Verification items for the finished model (mm, model axes). A direction names the side the tool comes from. Give positions to 0.01 mm unless a question says otherwise; leave off trailing zeros. Loops run counter-clockwise (first coordinate to the right, second up) from the corner with the lowest first, then second, coordinate; pieces in that order, holes last. Notation, with made-up numbers: (-30.5, -21) - (-14.5, -21) arc R9 ccw to (-14.5, -10) - close; hole circle Ø4 at (-7.5, -9.75). An arc over 180 degrees is marked (long way). Answer in a Markdown table with one row per item.
```python
from build123d import *

# Parameters (mm, degrees)
ESBO_O1_W                = 100
ESBO_O1_H                = 50
ESBO_O1_R                = 1
RESSALTO_EXTRUS_O1_DEPTH = 1.5
ESBO_O2_R                = 8.5
ESBO_O2_W                = 53
ESBO_O2_H                = 21
ESBO_O2_W_2              = 6
ESBO_O2_H_2              = 6
ESBO_O2_W_3              = 26.2
ESBO_O2_H_3              = 26.3
RESSALTO_EXTRUS_O4_DEPTH = 14.7
ESBO_O3_W                = 22.891769865
ESBO_O3_H                = 8.050029258
CORTE_EXTRUS_O1_DEPTH    = 9.7
ESBO_O4_R                = 3.5
RESSALTO_EXTRUS_O5_DEPTH = 17
ESBO_O5_W                = 55.7
ESBO_O5_H                = 43
RESSALTO_EXTRUS_O6_DEPTH = 18
ESBO_O6_W                = 26.2
ESBO_O6_H                = 14
RESSALTO_EXTRUS_O7_DEPTH = 0.2
ESBO_O7_W                = 26.2
ESBO_O7_H                = 10.560021921
CORTE_EXTRUS_O2_DEPTH    = 20.2


with BuildPart() as part:
    # Esboço1 → Ressalto-extrusão1 (new body)
    with BuildSketch(Plane(origin=(0, 0, 0), x_dir=(1, 0, 0), z_dir=(0, 1, 0))):
        Rectangle(ESBO_O1_W, ESBO_O1_H)
        with Locations(Location((43.75, 18.75, 0), (0, 0, 270))):
            Circle(ESBO_O1_R, mode=Mode.SUBTRACT)
        with Locations(Location((43.75, -18.75, 0), (0, 0, 270))):
            Circle(ESBO_O1_R, mode=Mode.SUBTRACT)
        with Locations(Location((-43.75, 18.749999801, 0), (0, 0, 270))):
            Circle(ESBO_O1_R, mode=Mode.SUBTRACT)
        with Locations(Location((-43.751173924, -18.750000181, 0), (0, 0, 270))):
            Circle(ESBO_O1_R, mode=Mode.SUBTRACT)
    extrude(amount=RESSALTO_EXTRUS_O1_DEPTH)

    # Esboço2 → Ressalto-extrusão4 (add)
    with BuildSketch(Plane(origin=(0, 1.5, 0), x_dir=(1, 0, 0), z_dir=(0, 1, 0))):
        with Locations(Location((33.5, -22.5, 0), (0, 0, 342.895364823))):
            Circle(ESBO_O2_R)
        with Locations(Location((-34.1, -22.5, 0), (0, 0, 197.104635177))):
            Circle(ESBO_O2_R)
        with Locations((-15.9, 5.5)):
            Rectangle(ESBO_O2_W, ESBO_O2_H)
        with Locations((22.3, 13)):
            Rectangle(ESBO_O2_W_2, ESBO_O2_H_2)
        with Locations((35.6, 13)):
            Rectangle(ESBO_O2_W_2, ESBO_O2_H_2)
        with Locations((-0.1, -19.15)):
            Rectangle(ESBO_O2_W_3, ESBO_O2_H_3)
    extrude(amount=RESSALTO_EXTRUS_O4_DEPTH)

    # Esboço3 → Corte-extrusão1 (cut)
    with BuildSketch(Plane(origin=(0, 16.2, 0), x_dir=(1, 0, 0), z_dir=(0, 1, 0))):
        with Locations((27.154115068, 14.025014629)):
            Rectangle(ESBO_O3_W, ESBO_O3_H)
    extrude(amount=-CORTE_EXTRUS_O1_DEPTH, mode=Mode.SUBTRACT)

    # Esboço4 → Ressalto-extrusão5 (add)
    with BuildSketch(Plane(origin=(0, 16.2, 0), x_dir=(1, 0, 0), z_dir=(0, 1, 0))):
        with Locations(Location((33.5, -22.5, 0), (0, 0, 270))):
            Circle(ESBO_O4_R)
        with Locations(Location((-34.1, -22.5, 0), (0, 0, 270))):
            Circle(ESBO_O4_R)
    extrude(amount=RESSALTO_EXTRUS_O5_DEPTH)

    # Esboço5 → Ressalto-extrusão6 (add)
    with BuildSketch(Plane.XZ):
        with Locations((-4.35, -5.5)):
            Rectangle(ESBO_O5_W, ESBO_O5_H)
    extrude(amount=RESSALTO_EXTRUS_O6_DEPTH)

    # Esboço6 → Ressalto-extrusão7 (add)
    with BuildSketch(Plane(origin=(0, 16.2, 0), x_dir=(1, 0, 0), z_dir=(0, 1, 0))):
        with Locations((-0.1, -17)):
            Rectangle(ESBO_O6_W, ESBO_O6_H)
    extrude(amount=RESSALTO_EXTRUS_O7_DEPTH)

    # Esboço7 → Corte-extrusão2 (cut)
    with BuildSketch(Plane.XY.offset(32.3)):
        with Locations((-0.1, 6.780010961)):
            Rectangle(ESBO_O7_W, ESBO_O7_H)
    extrude(amount=-CORTE_EXTRUS_O2_DEPTH, mode=Mode.SUBTRACT)


solid = part.part
```
Q1. Draft check along X on faces 6 (the face through (-16, 16.2, -6)), 7 (the face through (42, 8.7, 22.4)), 8 (the face through (-32.2, -9, -6)). Enter one of: +X half, -X half, draft (parallel to the pull), parting line (faces both ways), or undercut.
Completed:
| item | result |
|---|---|
| face 6 | draft |
| face 7 | undercut |
| face 8 | -X half |
Q2. Sectioned sample at B-B (z = 22.5). Record the cut outline in (x, y), and give its area (3 significant figures).
Completed:
| item | result |
|---|---|
| outline | (-50, 0) - (50, 0) - (50, 1.5) - (42, 1.5) - (42, 16.2) - (37, 16.2) - (37, 33.2) - (30, 33.2) - (30, 16.2) - (25, 16.2) - (25, 1.5) - (-25.6, 1.5) - (-25.6, 16.2) - (-30.6, 16.2) - (-30.6, 33.2) - (-37.6, 33.2) - (-37.6, 16.2) - (-42.6, 16.2) - (-42.6, 1.5) - (-50, 1.5) - close; (-13.2, 12.06) - (13, 12.06) - (13, 16.4) - (-13.2, 16.4) - close |
| area | 1,000 mm^2 |
Q3. Tool access check on faces 1 (the face through (-35, 1.5, 28)), 2 (the face through (0, 16.2, 8)), 3 (the face through (0, 16.4, 17)), 4 (the face through (-35.06, 16.2, 18.97)), 5 (the face through (0, 16.2, 28)). Record the directions out of +Z, -Z, +X, -X, +Y, -Y that give a thin tool (end or side, any length) a straight path to the whole face; none if there is none.
Completed:
| item | result |
|---|---|
| face 1 | +Z, +X, -X, -Y |
| face 2 | -Z, +X, -X, +Y |
| face 3 | +Z, -Z, +Y |
| face 4 | +Y |
| face 5 | +Z, +Y |
Q4. Thickness scan on line 1 (X direction, y = 0.85, z = 18.75); line 2 (Y direction, x = -8, z = 18); line 3 (Y direction, x = 41.5, z = 16). Record the ranges inside material, lowest first.
Completed:
| item | result |
|---|---|
| line 1 | -50 to -44.75, -42.75 to 42.75, 44.75 to 50 |
| line 2 | 0 to 1.5, 12.06 to 16.4 |
| line 3 | 0 to 1.5 |
Q5. Sectioned sample at C-C (z = -2.5). Record the cut outline in (x, y), and give its area (3 significant figures).
Completed:
| item | result |
|---|---|
| outline | (-50, 0) - (-32.2, 0) - (-32.2, -18) - (23.5, -18) - (23.5, 0) - (50, 0) - (50, 1.5) - (10.6, 1.5) - (10.6, 16.2) - (-42.4, 16.2) - (-42.4, 1.5) - (-50, 1.5) - close |
| area | 1,930 mm^2 |
Q6. Sectioned sample at A-A (y = 9). Record the cut outline in (x, z), and give its area (3 significant figures).
Completed:
| item | result |
|---|---|
| outline | circle Ø17 at (-34.1, 22.5); (-42.4, -16) - (10.6, -16) - (10.6, 5) - (-42.4, 5) - close; (-13.2, 6) - (13, 6) - (13, 12.1) - (-13.2, 12.1) - close; circle Ø17 at (33.5, 22.5) |
| area | 1,730 mm^2 |
Q7. Sectioned sample at D-D (y = 29). Record the cut outline in (x, z), and give its area (3 significant figures).
Completed:
| item | result |
|---|---|
| outline | circle Ø7 at (-34.1, 22.5); circle Ø7 at (33.5, 22.5) |
| area | 77.0 mm^2 |
Q8. Go/stop test with flat-tipped pins: P1, Ø1.5, axis at x = 15, z = 15.5, coming from the +Y side; P2, Ø18.5, axis at x = -36.5, z = 26, coming from the +Y side; P3, Ø6, axis at x = -6.5, z = 26.5, coming from the -Y side; P4, Ø2.5, axis at y = 4.5, z = -12.5, coming from the -X side. Record where each tip stops, or that it passes through.
Completed:
| item | result |
|---|---|
| P1 | y = 1.5 |
| P2 | y = 33.2 |
| P3 | y = 0 |
| P4 | x = -42.4 |
